For this review, take the finished solid that the model builds, in its own axes (mm). A direction names the side the tool comes from. Round coordinates to 2 decimals unless told otherwise and drop trailing zeros. Order: outer loops, then holes, each group sorted by start corner. A loop starts at its lowest first (then second) coordinate and runs counter-clockwise, first axis right, second up. Notation, with made-up numbers: M 56.25,11.5 L 70.25,11.5 A28 ccw 70.25,32.5 Z; hole C 5.25,78.25 d1. An arc over 180 degrees is marked long. Write item = value, one per line. Start each with the question number.
from build123d import *

# Parameters (mm, degrees)
SKETCH_1_W           = 19
SKETCH_1_H           = 19
SKETCH_1_W_2         = 55
SKETCH_1_H_2         = 7
EXTRUDE_1_DEPTH      = 21
SKETCH_1_3_W         = 13
SKETCH_1_3_H         = 13
CUT_EXTRUDE_1_DEPTH  = 21
SKETCH_1_12_W        = 19
SKETCH_1_12_H        = 19
SKETCH_1_12_W_2      = 14.6
SKETCH_1_12_H_2      = 14.6
CUT_EXTRUDE_6_DEPTH  = 18
CUT_EXTRUDE_7_DEPTH  = 14.5
SKETCH_4_W           = 3.5
SKETCH_4_H           = 7
SKETCH_4_W_2         = 3.504900739
EXTRUDE_2_DEPTH      = 27.5
CUT_EXTRUDE_9_DEPTH  = 2
SKETCH_7_W           = 3.6
SKETCH_7_H           = 3.966529086
CUT_EXTRUDE_10_DEPTH = 2
SKETCH_9_W           = 3.6
SKETCH_9_H           = 3.966529086
CUT_EXTRUDE_11_DEPTH = 2
SKETCH_10_W          = 3.6
SKETCH_10_H          = 3.966529086
CUT_EXTRUDE_12_DEPTH = 2


with BuildPart() as part:
    # Sketch 1 → Extrude 1 (new body, symmetric)
    with BuildSketch(Plane.XY):
        Rectangle(SKETCH_1_W, SKETCH_1_H)
        with Locations((0, -13)):
            Rectangle(SKETCH_1_W_2, SKETCH_1_H_2)
    extrude(amount=EXTRUDE_1_DEPTH, both=True)

    # Sketch 1_3 → Cut-Extrude 1 (cut, symmetric)
    with BuildSketch(Plane.XY):
        Rectangle(SKETCH_1_3_W, SKETCH_1_3_H)
    extrude(amount=CUT_EXTRUDE_1_DEPTH, both=True, mode=Mode.SUBTRACT)

    # Sketch 1_12 → Cut-Extrude 6 (cut, symmetric)
    with BuildSketch(Plane.XY):
        Rectangle(SKETCH_1_12_W, SKETCH_1_12_H)
        Rectangle(SKETCH_1_12_W_2, SKETCH_1_12_H_2, mode=Mode.SUBTRACT)
    extrude(amount=CUT_EXTRUDE_6_DEPTH, both=True, mode=Mode.SUBTRACT)

    # Sketch 1_13 → Cut-Extrude 7 (cut, symmetric)
    with BuildSketch(Plane.XY):
        Polygon((9.5, -9.5), (-9.5, -9.5), (-27.5, -9.5), (-27.5, -16.5), (27.5, -16.5), (27.5, -9.5), align=None)
    extrude(amount=CUT_EXTRUDE_7_DEPTH, both=True, mode=Mode.SUBTRACT)

    # Sketch 4 → Extrude 2 (add, symmetric)
    with BuildSketch(Plane(origin=(0, 0, 0), x_dir=(0, 0, -1), z_dir=(1, 0, 0))):
        with Locations((22.75, -13)):
            Rectangle(SKETCH_4_W, SKETCH_4_H)
        with Locations((-22.752450369, -13)):
            Rectangle(SKETCH_4_W_2, SKETCH_4_H)
    extrude(amount=EXTRUDE_2_DEPTH, both=True)

    # Sketch 5 → Cut-Extrude 9 (cut)
    with BuildSketch(Plane(origin=(0, 0, -24.5), x_dir=(-1, 0, 0), z_dir=(0, 0, -1))):
        Polygon((-27.5, -9.5), (-27.5, -16.5), (-24.66, -16.5), (-24.66, -12.503647236), (-22.86, -12.503647236), (-21.06, -12.503647236), (-21.06, -16.5), (-19.58, -16.5), (-19.58, -12.503647236), (-17.78, -12.503647236), (-15.98, -12.503647236), (-15.98, -16.5), (-14.5, -16.5), (-14.5, -12.503647236), (-12.7, -12.503647236), (-10.9, -12.503647236), (-10.9, -16.5), (-9.42, -16.5), (-9.42, -12.503647236), (-7.62, -12.503647236), (-5.82, -12.503647236), (-5.82, -16.5), (-4.34, -16.5), (-4.34, -12.511103156), (-0.74, -12.511103156), (-0.74, -16.5), (0.731971317, -16.5), (0.731971317, -12.518559075), (2.535985659, -12.518559075), (4.34, -12.518559075), (4.34, -16.5), (7.62, -16.5), (10.896293739, -16.5), (10.896293739, -12.507758798), (12.698146869, -12.507758798), (14.5, -12.507758798), (14.5, -16.5), (15.980045705, -16.5), (15.980045705, -12.508203705), (17.780055728, -12.508203705), (19.580065752, -12.508203705), (19.580065752, -16.5), (21.06, -16.5), (21.06, -12.508203705), (22.859139551, -12.508203705), (24.658279102, -12.508203705), (24.658279102, -16.5), (27.5, -16.5), (27.5, -9.5), (9.5, -9.5), (-9.5, -9.5), align=None)
        Polygon((9.42, -16.487143942), (7.62, -16.487143942), (5.82, -16.487143942), (5.82, -12.520614856), (7.62, -12.520614856), (9.42, -12.520614856), align=None, mode=Mode.SUBTRACT)
    extrude(amount=-CUT_EXTRUDE_9_DEPTH, mode=Mode.SUBTRACT)

    # Sketch 7 → Cut-Extrude 10 (cut)
    with BuildSketch(Plane(origin=(0, 0, 14.5), x_dir=(-1, 0, 0), z_dir=(0, 0, -1))):
        Polygon((19.580065752, -16.5), (21.06, -16.5), (21.06, -12.508203705), (24.658279102, -12.508203705), (24.658279102, -16.5), (27.5, -16.5), (27.5, -9.5), (-27.5, -9.5), (-27.5, -16.5), (-24.66, -16.5), (-24.66, -12.503647236), (-21.06, -12.503647236), (-21.06, -16.5), (-19.58, -16.5), (-19.58, -12.503647236), (-15.98, -12.503647236), (-15.98, -16.5), (-14.5, -16.5), (-14.5, -12.503647236), (-10.9, -12.503647236), (-10.9, -16.5), (-9.42, -16.5), (-9.42, -12.503647236), (-5.82, -12.503647236), (-5.82, -16.5), (-4.34, -16.5), (-4.34, -12.511103156), (-0.74, -12.511103156), (-0.74, -16.5), (0.731971317, -16.5), (0.731971317, -12.518559075), (4.34, -12.518559075), (4.34, -16.5), (10.896293739, -16.5), (10.896293739, -12.507758798), (14.5, -12.507758798), (14.5, -16.5), (15.980045705, -16.5), (15.980045705, -12.508203705), (19.580065752, -12.508203705), align=None)
        with Locations((7.62, -14.503879399)):
            Rectangle(SKETCH_7_W, SKETCH_7_H, mode=Mode.SUBTRACT)
    extrude(amount=-CUT_EXTRUDE_10_DEPTH, mode=Mode.SUBTRACT)

    # Sketch 9 → Cut-Extrude 11 (cut)
    with BuildSketch(Plane.XY.offset(-14.5)):
        Polygon((24.66, -16.5), (27.5, -16.5), (27.5, -9.5), (-27.5, -9.5), (-27.5, -16.5), (-24.658279102, -16.5), (-24.658279102, -12.508203705), (-21.06, -12.508203705), (-21.06, -16.5), (-19.580065752, -16.5), (-19.580065752, -12.508203705), (-15.980045705, -12.508203705), (-15.980045705, -16.5), (-14.5, -16.5), (-14.5, -12.507758798), (-10.896293739, -12.507758798), (-10.896293739, -16.5), (-4.34, -16.5), (-4.34, -12.518559075), (-0.731971317, -12.518559075), (-0.731971317, -16.5), (0.74, -16.5), (0.74, -12.511103156), (4.34, -12.511103156), (4.34, -16.5), (5.82, -16.5), (5.82, -12.503647236), (9.42, -12.503647236), (9.42, -16.5), (10.9, -16.5), (10.9, -12.503647236), (14.5, -12.503647236), (14.5, -16.5), (15.98, -16.5), (15.98, -12.503647236), (19.58, -12.503647236), (19.58, -16.5), (21.06, -16.5), (21.06, -12.503647236), (24.66, -12.503647236), align=None)
        with Locations((-7.62, -14.503879399)):
            Rectangle(SKETCH_9_W, SKETCH_9_H, mode=Mode.SUBTRACT)
    extrude(amount=-CUT_EXTRUDE_11_DEPTH, mode=Mode.SUBTRACT)

    # Sketch 10 → Cut-Extrude 12 (cut)
    with BuildSketch(Plane.XY.offset(24.504900739)):
        Polygon((27.5, -9.5), (-27.5, -9.5), (-27.5, -16.5), (-24.658279102, -16.5), (-24.658279102, -12.508203705), (-21.06, -12.508203705), (-21.06, -16.5), (-19.580065752, -16.5), (-19.580065752, -12.508203705), (-15.980045705, -12.508203705), (-15.980045705, -16.5), (-14.5, -16.5), (-14.5, -12.507758798), (-10.896293739, -12.507758798), (-10.896293739, -16.5), (-4.34, -16.5), (-4.34, -12.518559075), (-0.731971317, -12.518559075), (-0.731971317, -16.5), (0.74, -16.5), (0.74, -12.511103156), (4.34, -12.511103156), (4.34, -16.5), (5.82, -16.5), (5.82, -12.503647236), (9.42, -12.503647236), (9.42, -16.5), (10.9, -16.5), (10.9, -12.503647236), (14.5, -12.503647236), (14.5, -16.5), (15.98, -16.5), (15.98, -12.503647236), (19.58, -12.503647236), (19.58, -16.5), (21.06, -16.5), (21.06, -12.503647236), (24.66, -12.503647236), (24.66, -16.5), (27.5, -16.5), align=None)
        with Locations((-7.62, -14.503879399)):
            Rectangle(SKETCH_10_W, SKETCH_10_H, mode=Mode.SUBTRACT)
    extrude(amount=-CUT_EXTRUDE_12_DEPTH, mode=Mode.SUBTRACT)


solid = part.part
(1) For faces 1 (the flat face through (18, -14, 14.5)), 2 (the flat face through (9.5, 0, 20)), list the 3-axis set-ups (+Z, -Z, +X, -X, +Y, -Y) from which the entire face can be reached by the end or side of a thin tool; tool diameter is ignored.
(2) Draft analysis for pull direction Z (two halves, no side actions). For faces 3 (the flat face through (-18, -15, -24.5)), 4 (the flat face through (13, -12.504, -15)), 5 (the flat face through (-15.98, -14, 24)), state which applies: released by +Z, released by -Z, zero draft, split by the parting line, or undercut.
(3) We need section C-C, the plane z = 20. Write out the cut boundary in (x, y).
(4) We need section A-A, the plane x = 12.5. Write out the cut boundary in (y, z).
(5) Insertion check: pin 1 (1.6 mm diameter, centred on y = -14.5, z = 15.5, fed in from -X); pin 2 (0.6 mm diameter, centred on x = -23, z = 15, fed in from +Y); pin 3 (1 mm diameter, centred on y = 1.5, z = 8, fed in from -X); pin 4 (8 mm diameter, centred on y = -12.5, z = 4, fed in from +X). Each pin has a flat end and moves straight along its axis. Give the tip position at first contact, or say it passes through.
(6) For line 1 along X through (y, z) = (1, -1); line 2 along Z through (x, y) = (-20, -12), list the stretches that pass through material, from the lowest coordinate up.
(7) We need section B-B, the plane y = -8.75. Write out the cut boundary in (x, z).
(8) We need section D-D, the plane z = -2. Write out the cut boundary in (x, y).
Values:
q1.face_1 = +X, -X, +Y, -Y
q1.face_2 = +Z, -Z, +X, +Y
q2.face_3 = released by -Z
q2.face_4 = undercut
q2.face_5 = zero draft
q3.outline = M -27.5,-16.5 L 27.5,-16.5 L 27.5,-9.5 L 9.5,-9.5 L 9.5,9.5 L -9.5,9.5 L -9.5,-9.5 L -27.5,-9.5 Z; hole M -6.5,-6.5 L 6.5,-6.5 L 6.5,6.5 L -6.5,6.5 Z
q4.outline = M -16.5,-24.5 L -12.5,-24.5 L -12.5,-22.5 L -9.5,-22.5 L -9.5,-16.5 L -12.5,-16.5 L -12.5,-14.5 L -16.5,-14.5 Z; M -16.5,14.5 L -12.5,14.5 L -12.5,16.5 L -9.5,16.5 L -9.5,22.5 L -12.5,22.5 L -12.5,24.5 L -16.5,24.5 Z
q5.pin_1 = -24.66
q5.pin_2 = -12.51
q5.pin_3 = -7.3
q5.pin_4 = through
q6.line_1 = -7.3 to -6.5, 6.5 to 7.3
q6.line_2 = -22.5 to -16.5, 16.5 to 22.5
q7.outline = M -9.5,-21 L 9.5,-21 L 9.5,-18 L -9.5,-18 Z; M -9.5,18 L 9.5,18 L 9.5,21 L -9.5,21 Z
q8.outline = M -7.3,-7.3 L 7.3,-7.3 L 7.3,7.3 L -7.3,7.3 Z; hole M -6.5,-6.5 L 6.5,-6.5 L 6.5,6.5 L -6.5,6.5 Z
